from build123d import *

# Parameters (mm, degrees)
F0_W     = 14
F0_H     = 11
F0_W_2   = 4
F0_H_2   = 7
F1_DEPTH = 2
F2_SIZE  = 0.4


with BuildPart() as f1:
    # F0 (on Top) → F1 (new body)
    with BuildSketch(Plane.XY):
        with Locations((3.093662, 1.61453)):
            Rectangle(F0_W, F0_H)
        with Locations((0.093662, 1.61453)):
            Rectangle(F0_W_2, F0_H_2, mode=Mode.SUBTRACT)
        with Locations((6.093662, 1.61453)):
            Rectangle(F0_W_2, F0_H_2, mode=Mode.SUBTRACT)
    extrude(amount=F1_DEPTH)

    # F2
    f2_edges = [f1.edges().sort_by_distance(p)[0] for p in [
        (3.093662, -3.88547, 2),
        (-3.906338, 1.61453, 2),
        (-1.906338, 1.61453, 2),
        (2.093662, 1.61453, 2),
        (4.093662, 1.61453, 2),
        (8.093662, 1.61453, 2),
        (0.093662, 5.11453, 2),
        (0.093662, -1.88547, 2),
        (6.093662, -1.88547, 2),
        (10.093662, 1.61453, 2),
        (3.093662, 7.11453, 2),
        (6.093662, 5.11453, 2),
        (10.093662, 7.11453, 1),
        (-3.906338, 7.11453, 1),
        (10.093662, -3.88547, 1),
        (-3.906338, -3.88547, 1),
        (3.093662, -3.88547, 0),
        (10.093662, 1.61453, 0),
        (8.093662, 1.61453, 0),
        (6.093662, 5.11453, 0),
        (4.093662, 1.61453, 0),
        (6.093662, -1.88547, 0),
        (2.093662, 1.61453, 0),
        (0.093662, 5.11453, 0),
        (0.093662, -1.88547, 0),
        (-1.906338, 1.61453, 0),
        (-3.906338, 1.61453, 0),
        (3.093662, 7.11453, 0),
    ]]
    chamfer(f2_edges, length=F2_SIZE)


solid = f1.part
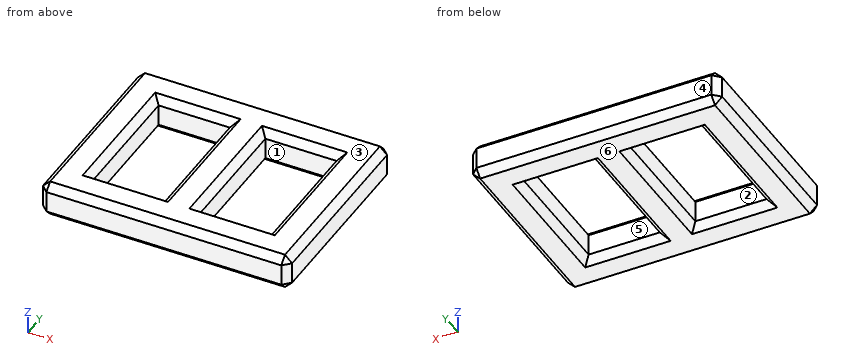
Can you work these out from the model? Positions are in its coordinate system, mm. Face numbers are marked on the shaded views. A direction names the side the tool comes from. Give positions to 0.01 mm unless a question says otherwise; leave off trailing zeros. Loops run counter-clockwise (first coordinate to the right, second up) from the corner with the lowest first, then second, coordinate; pieces in that order, holes last. Notation, with made-up numbers: M 54,36 L 90,36 A22 cw 90,55 Z; hole C 86,61 d8. An arc over 180 degrees is marked long. One line per item, written item: value. Start each with the question number.
1) Thinking about a two-plate mould opening in Y: for the marked faces 1, 2, 3 and 4, which applies, +Y half, -Y half, draft (parallel to the pull), parting line (faces both ways), or undercut?
2) If I drill on line 1 (X direction, y = 2, z = 0.6); line 2 (Y direction, x = 4.75, z = 1.5); line 3 (X direction, y = 1.5, z = 0.25), over which ranges is the centre line in solid material (lowest first)? Write a range as [from, to].
3) On a 3-axis mill with a long thin cutter (end or side, diameter ignored), from which of +Z, -Z, +X, -X, +Y, -Y can I reach the whole of each face in a straight line? I mean the marked faces 5 and 6. Say none if no direction works.
4) If we section it at A-A, the plane x = -0.5: Write out the boundary of the cut face in (y, z), and give its area (3 significant figures).
5) If we section it at C-C, the plane z = 0.7: Write out the boundary of the cut face in (x, y).
6) If we section it at B-B, the plane y = 2.75: Write out the boundary of the cut face in (x, z).
7) I'm going to push a flat-ended pin straight in: pin 1 (2 mm diameter, centred on x = 0, y = 0, fed in from -Z). Where does the tip first touch, or does it pass through?
Completed:
1. face 1: undercut
1. face 2: undercut
1. face 3: draft
1. face 4: +Y half
2. line 1: x = [-3.91, -1.91], [2.09, 4.09], [8.09, 10.09]
2. line 2: y = [-3.89, -1.89], [5.11, 7.11]
2. line 3: x = [-3.76, -2.06], [2.24, 3.94], [8.24, 9.94]
3. face 5: +Z, -Z
3. face 6: -Z, +X, -X, +Y, -Y
4. outline: M -3.89,0.4 L -3.49,0 L -2.29,0 L -1.89,0.4 L -1.89,1.6 L -2.29,2 L -3.49,2 L -3.89,1.6 Z; M 5.11,0.4 L 5.51,0 L 6.71,0 L 7.11,0.4 L 7.11,1.6 L 6.71,2 L 5.51,2 L 5.11,1.6 Z
4. area: 7.36 mm^2
5. outline: M -3.91,-3.49 L -3.51,-3.89 L 9.69,-3.89 L 10.09,-3.49 L 10.09,6.71 L 9.69,7.11 L -3.51,7.11 L -3.91,6.71 Z; hole M -1.91,-1.89 L 2.09,-1.89 L 2.09,5.11 L -1.91,5.11 Z; hole M 4.09,-1.89 L 8.09,-1.89 L 8.09,5.11 L 4.09,5.11 Z
6. outline: M -3.91,0.4 L -3.51,0 L -2.31,0 L -1.91,0.4 L -1.91,1.6 L -2.31,2 L -3.51,2 L -3.91,1.6 Z; M 2.09,0.4 L 2.49,0 L 3.69,0 L 4.09,0.4 L 4.09,1.6 L 3.69,2 L 2.49,2 L 2.09,1.6 Z; M 8.09,0.4 L 8.49,0 L 9.69,0 L 10.09,0.4 L 10.09,1.6 L 9.69,2 L 8.49,2 L 8.09,1.6 Z
7. pin 1: passes through
